The listing builds one solid part. Answer for the finished solid, in the listing's coordinates (mm). A direction names the side the tool comes from. Round coordinates to 2 decimals unless told otherwise and drop trailing zeros. Loops run counter-clockwise (first coordinate to the right, second up) from the corner with the lowest first, then second, coordinate; pieces in that order, holes last. Notation, with made-up numbers: M -29,44.5 L 22,44.5 A25 ccw 22,71.5 Z; hole C 20.25,-1 d5. An arc over 180 degrees is marked long. Answer as a JSON object with one key per item and string values.
```python
from build123d import *

# Parameters (mm, degrees)
SKETCH1_W           = 101.6
SKETCH1_H           = 50.8
SKETCH1_W_2         = 88.9
SKETCH1_H_2         = 38.1
BOSS_EXTRUDE1_DEPTH = 457.2
SKETCH4_W           = 25.4
SKETCH4_H           = 50.8
BOSS_EXTRUDE3_DEPTH = 0.0254


with BuildPart() as part:
    # Sketch1 → Boss-Extrude1 (new body, symmetric)
    with BuildSketch(Plane.XY):
        Rectangle(SKETCH1_W, SKETCH1_H)
        Rectangle(SKETCH1_W_2, SKETCH1_H_2, mode=Mode.SUBTRACT)
    extrude(amount=BOSS_EXTRUDE1_DEPTH, both=True)

    # Sketch4 → Boss-Extrude3 (add)
    with BuildSketch(Plane.ZY.offset(50.8)):
        Rectangle(SKETCH4_W, SKETCH4_H)
    extrude(amount=BOSS_EXTRUDE3_DEPTH)


solid = part.part
```
Item 1: A flat-ended cylindrical pin translates along its axis: P1, Ø5, axis at y = 6.5, z = 261.5, coming from the -X side. Find the tip coordinate at first contact, or state that the pin passes through.
Values follow:
{"P1": "x = -50.8"}
Item 2: Which of the six approach directions +Z, -Z, +X, -X, +Y, -Y give full straight-line access (tool end or side, diameter ignored) to faces 4 (the face through (44.45, 0, 6)), 5 (the face through (-50.8, 0, 238))?
Values follow:
{"face 4": "+Z, -Z", "face 5": "+Z, -Z, -X, +Y, -Y"}
Item 3: The part is cut by section B-B (x = -31). Give the vertices of the cut face in (y, z).
Values follow:
{"outline": "M -25.4,-457.2 L -19.05,-457.2 L -19.05,457.2 L -25.4,457.2 Z; M 19.05,-457.2 L 25.4,-457.2 L 25.4,457.2 L 19.05,457.2 Z"}
Item 4: The part is cut by section C-C (z = 140.5). Give the vertices of the cut face in (x, y).
Values follow:
{"outline": "M -50.8,-25.4 L 50.8,-25.4 L 50.8,25.4 L -50.8,25.4 Z; hole M -44.45,-19.05 L 44.45,-19.05 L 44.45,19.05 L -44.45,19.05 Z"}
Item 5: Determine the mould class of faces 1 (the face through (-50.8, 0, -232)), 2 (the face through (-1, 25.4, 6)), 3 (the face through (-1, 19.05, 6)) for opening direction Y: released by +Y, released by -Y, zero draft, split by the parting line, or undercut.
Values follow:
{"face 1": "zero draft", "face 2": "released by +Y", "face 3": "undercut"}
Item 6: Straight lines are drawn through the part: line 1 (Y direction, x = 9, z = -133); line 2 (X direction, y = -4, z = 405); line 3 (X direction, y = 21.5, z = 265.5). For each, find the intervals that lie inside material, in ascending order.
Values follow:
{"line 1": "-25.4 to -19.05, 19.05 to 25.4", "line 2": "-50.8 to -44.45, 44.45 to 50.8", "line 3": "-50.8 to 50.8"}
